Could you check a few things on this model? Use its own coordinates, in mm. Coordinates: 2 decimals unless noted, no trailing zeros. Write each loop counter-clockwise with the first axis right and the second up, starting at its lowest first coordinate (ties: lowest second). Pieces come first, ordered by that corner, then holes. Notation, with made-up numbers: M -9.5,43.5 L 43.5,43.5 A22 ccw 43.5,51.5 Z; hole C -32,58.5 d1. An arc over 180 degrees is marked long. Write item = value, one per line.
```python
from build123d import *
from build123d.topology import SkipClean

# Parameters (mm, degrees)
STOCK_FRAME_START          = -95
STOCK_FRAME_MASTER_1_DEPTH = 5


# Read off the part's stored shape, not the designer's step: Stock-Frame master-1
with BuildPart() as part:
    # Stock-Frame master-1 outline → Stock-Frame master-1 (new body)
    with BuildSketch(Plane(origin=(0, 0, 0), x_dir=(1, 0, 0), z_dir=(0, 1, 0)).offset(STOCK_FRAME_START)):
        with BuildLine():
            Line((48.103357378, 83.317458993), (0, 0))
            Line((0, 0), (165.5, 0))
            ThreePointArc((165.5, 0), (167.5, 2), (169.5, 0))
            Line((169.5, 0), (177.5, 0))
            Line((177.5, 0), (177.5, 16.693176311))
            ThreePointArc((177.5, 16.693176311), (176.227241336, 21.443176311), (172.75, 24.920417647))
            Line((172.75, 24.920417647), (53.978357378, 93.493257487))
            Line((53.978357378, 93.493257487), (50.103357378, 86.781560608))
            ThreePointArc((50.103357378, 86.781560608), (50.835408185, 84.049509801), (48.103357378, 83.317458993))
        make_face()
    extrude(amount=STOCK_FRAME_MASTER_1_DEPTH)

    # Mirror1: part across plane


with BuildPart() as part_1:
    with SkipClean():  # the faces are left unmerged after this step: merging them gives an invalid solid
        add(part.part)
        add(part.part.mirror(Plane(origin=(220, -90, 0), x_dir=(1, 0, 0), z_dir=(0, 0, -1))))


with BuildPart() as body_2:
    # Mirror2: mirrored copy
    add(part_1.part.mirror(Plane(origin=(0, -90, 0), x_dir=(-0.49999999999999406, 0, 0.866025403784442), z_dir=(0.8660254037844419, 0, 0.4999999999999941))))


with BuildPart() as part_2:
    with SkipClean():  # the faces are left unmerged after this step: merging them gives an invalid solid
        add(part_1.part)

        # Mirror3: part across plane
        add(part_1.part.mirror(Plane(origin=(0, -90, 0), x_dir=(0.49999999999999406, 0, 0.866025403784442), z_dir=(0.8660254037844419, 0, -0.4999999999999941))))


with BuildPart() as body_2_1:
    add(body_2.part)

    # Combine1: union part
    add(part_2.part)


solid = body_2_1.part
```
Item 1: Imagine slicing it at B-B (z = -78). Write out the boundary of the cut face in (x, y), and give its area (3 significant figures).
Numbers:
outline = M -107.96,-95 L 80.81,-95 L 80.81,-90 L -107.96,-90 Z
area = 944 mm²
Item 2: Imagine slicing it at C-C (x = -31). Write out the boundary of the cut face in (y, z).
Numbers:
outline = M -95,-142.56 L -90,-142.56 L -90,142.56 L -95,142.56 Z
Item 3: I'm going to push flat-ended pins straight in: P1, Ø2, axis at x = -66, y = -94.5, coming from the +Z side; P2, Ø1.5, axis at x = -54.5, y = -91.5, coming from the +Z side. Where does each tip first touch, or does it pass through?
Numbers:
P1 = 162.99
P2 = 156.56
Item 4: Imagine slicing it at A-A (y = -93.1). Write out the boundary of the cut face in (x, z), and give its area (3 significant figures).
Numbers:
outline = M -107.96,-137.15 A9.5 ccw -103.21,-145.37 L -74.29,-162.07 A9.5 ccw -64.79,-162.07 L 172.75,-24.92 A9.5 ccw 177.5,-16.69 L 177.5,16.69 A9.5 ccw 172.75,24.92 L -64.79,162.07 A9.5 ccw -74.29,162.07 L -103.21,145.37 A9.5 ccw -107.96,137.15 Z; hole C -98.21,0 d4; hole C -83.75,-145.06 d4; hole C -83.75,145.06 d4; hole C 49.1,-85.05 d4; hole C 49.1,85.05 d4; hole C 167.5,0 d4
area = 57,900 mm²
